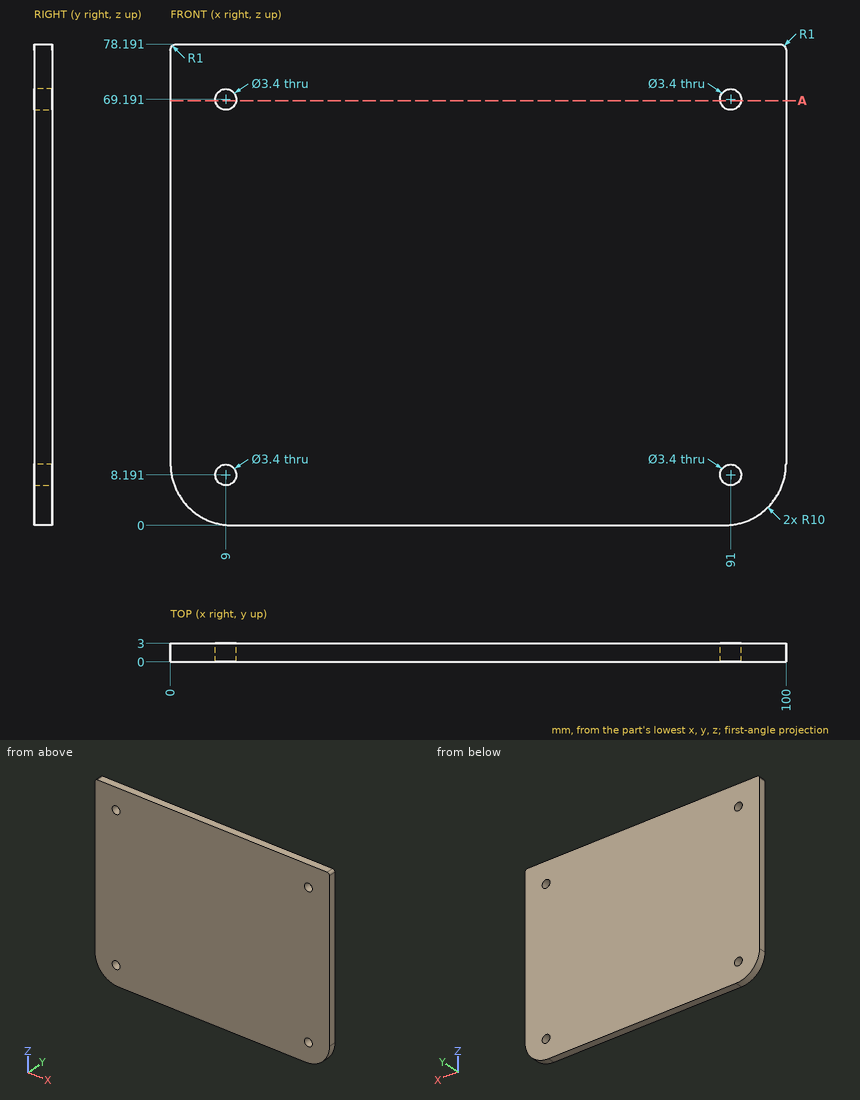
Can you work these out from the drawing? Everything is in mm from the part's minimum corner. Coordinates: 2 decimals unless noted, no trailing zeros. Loops run counter-clockwise (first coordinate to the right, second up) from the corner with the lowest first, then second, coordinate; pieces in that order, holes last.
1) For pin 1 (1 mm diameter, centred on x = 53.5, y = 2.5, fed in from -Z); pin 2 (2 mm diameter, centred on x = 91, z = 69.19, fed in from +Y); pin 3 (1 mm diameter, centred on y = 1, z = 9, fed in from -X), each with a flat end and sliding along its axis, tell me the tip position at first contact or that it passes through.
2) Imagine slicing it at A-A on z = 69. List the corners of the cut face in (x, y) for me.
3) I need wall thicknesses on probe 1 along Z at (x, y) = (91, 1.55). Which ranges of the line are inside material? Lowest first, please.
Completed:
1. pin 1: stops at z = 0
1. pin 2: passes through
1. pin 3: stops at x = 0.01
2. outline: (0, 0) - (7.31, 0) - (7.31, 3) - (0, 3) - close; (10.69, 0) - (89.31, 0) - (89.31, 3) - (10.69, 3) - close; (92.69, 0) - (100, 0) - (100, 3) - (92.69, 3) - close
3. probe 1: z = 0.05 to 6.49, 9.89 to 67.49, 70.89 to 78.19
